The drawing under review shows one solid part. Ordinate dimensions are in mm from its lowest x, y, z. A direction names the side the tool comes from. Coordinates: 2 decimals unless noted, no trailing zeros. Loops run counter-clockwise (first coordinate to the right, second up) from the corner with the lowest first, then second, coordinate; pieces in that order, holes last.
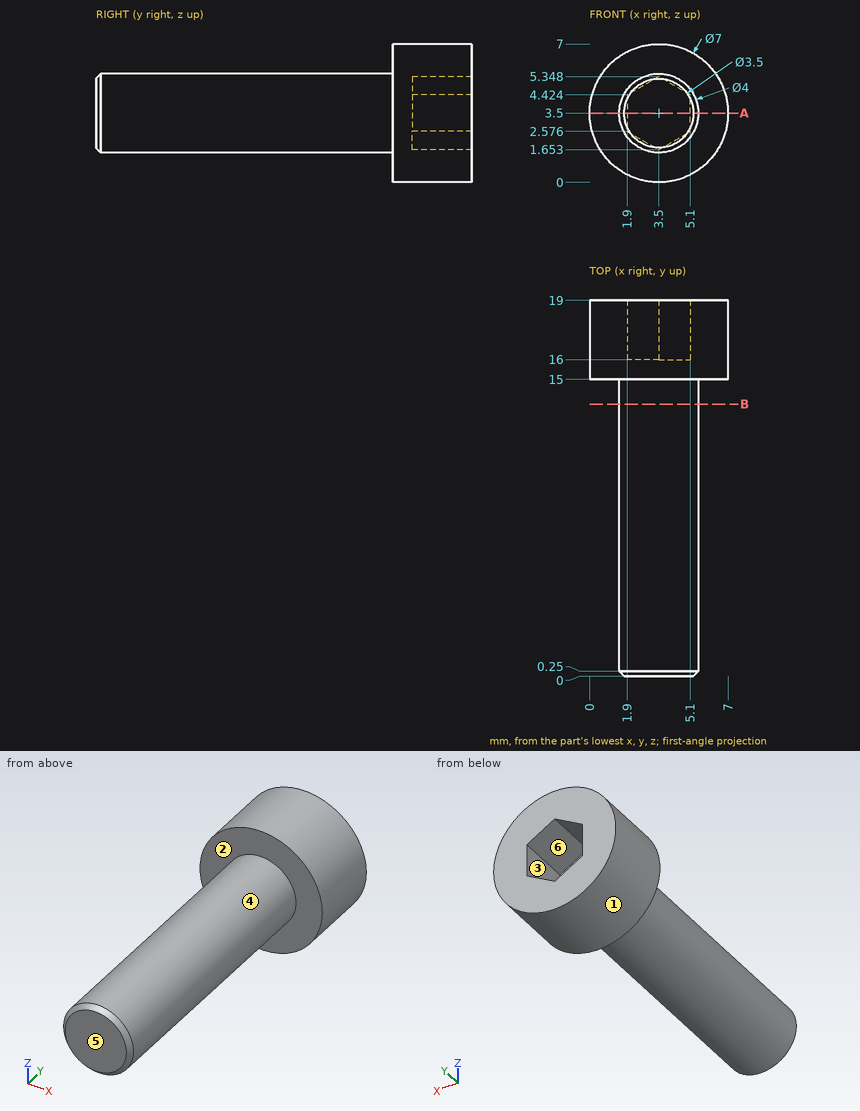
Q1. Take a section at A-A, the plane z = 3.5. Write out the cut boundary in (x, y).
Q2. Clearance check with flat-ended pins moving along their axes: pin 1 Ø3 at (y, z) = (4, 6) entering from -X; pin 2 Ø2 at (y, z) = (12.5, 4) entering from +X; pin 3 Ø3 at (x, y) = (6, 4.5) entering from -Z. State where each tip first meets the part, or that it passes through.
Q3. Take a section at B-B, the plane y = 13.75. Write out the cut boundary in (x, z), then the cut area to 3 significant figures.
Q4. For line 1 (Y direction, x = 3.75, z = 4); line 2 (Y direction, x = 5, z = 5); line 3 (Z direction, x = 3, y = 17.25) (1 decimal), list the stretches that pass through material, from the lowest coordinate up.
Q5. The part is to be moulded in two halves that separate along X. For the marked faces 3, 4, 5 and 6, say which applies: pulls with the +X half, pulls with the -X half, needs draft (parallel to the pull), parting line crosses it, or undercut.
Q6. Machinability: for the marked faces 1 and 2, which of the approach directions +Z, -Z, +X, -X, +Y, -Y give a long, thin tool a straight path to every point of the face, cutting with its end or side? Answer none if there is none.
Entries:
1. outline: (0, 15) - (1.5, 15) - (1.5, 0.25) - (1.75, 0) - (5.25, 0) - (5.5, 0.25) - (5.5, 15) - (7, 15) - (7, 19) - (5.1, 19) - (5.1, 16) - (1.9, 16) - (1.9, 19) - (0, 19) - close
2. pin 1: stops at x = 1.77
2. pin 2: stops at x = 5.5
2. pin 3: stops at z = 1.77
3. outline: circle Ø4 at (3.5, 3.5)
3. area: 12.6 mm2
4. line 1: y = 0 to 16
4. line 2: y = 15 to 19
4. line 3: z = 0 to 1.9, 5.1 to 7
5. face 3: undercut
5. face 4: parting line crosses it
5. face 5: needs draft
5. face 6: undercut
6. face 1: +Y, -Y
6. face 2: -Y
